The drawing under review shows one solid part. Ordinate dimensions are in mm from its lowest x, y, z. Coordinates: 2 decimals unless noted, no trailing zeros. Order: outer loops, then holes, each group sorted by start corner. A loop starts at its lowest first (then second) coordinate and runs counter-clockwise, first axis right, second up. Notation, with made-up numbers: (-34.5, 77.5) - (-28.5, 77.5) arc R27 ccw to (-28.5, 113.5) - close; hole circle Ø10 at (39.25, 50.5). An arc over 180 degrees is marked (long way). Answer in a Markdown table with one row per item.
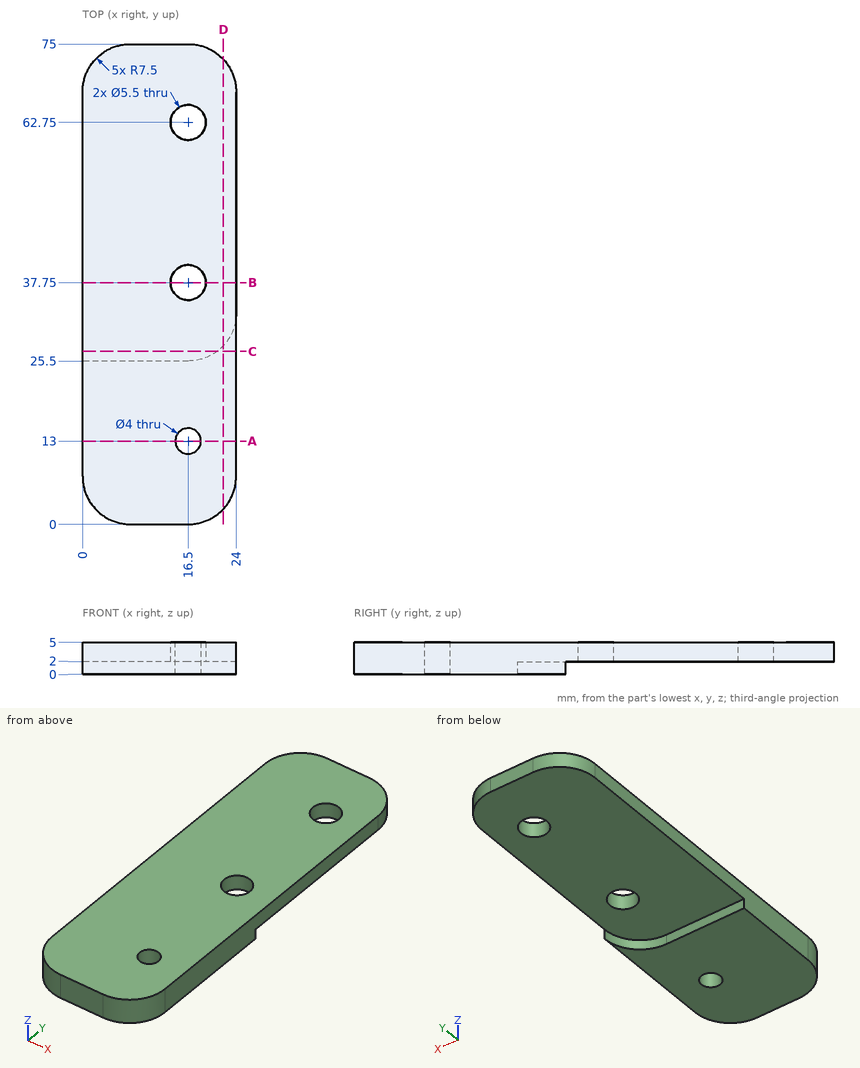
Item 1: Clearance check with flat-ended pins moving along their axes: pin 1 Ø6 at (x, y) = (10.5, 43) entering from -Z; pin 2 Ø0.6 at (x, z) = (6.5, 1.5) entering from +Y; pin 3 Ø3 at (x, z) = (21.5, 1.5) entering from -Y. State where each tip first meets the part, or that it passes through.
Check values:
| item | result |
|---|---|
| pin 1 | z = 2 |
| pin 2 | y = 25.5 |
| pin 3 | y = 0.87 |
Item 2: We need section A-A, the plane y = 13. Write out the cut boundary in (x, z), then the cut area to 3 significant figures.
Check values:
| item | result |
|---|---|
| outline | (0, 0) - (14.5, 0) - (14.5, 5) - (0, 5) - close; (18.5, 0) - (24, 0) - (24, 5) - (18.5, 5) - close |
| area | 100 mm^2 |
Item 3: We need section D-D, the plane x = 22. Write out the cut boundary in (y, z), then the cut area to 3 significant figures.
Check values:
| item | result |
|---|---|
| outline | (2.4, 0) - (27.9, 0) - (27.9, 2) - (72.6, 2) - (72.6, 5) - (2.4, 5) - close |
| area | 262 mm^2 |
Item 4: To check wall thickness, follow line 1 (X direction, y = 62.75, z = 2.75); line 2 (Z direction, x = 3, y = 69.5); line 3 (Y direction, x = 6.75, z = 4.1). State the ranges of each line that lie inside material, in increasing order. Write a range as from..to.
Check values:
| item | result |
|---|---|
| line 1 | 0..13.75, 19.25..24 |
| line 2 | 2..5 |
| line 3 | 0.04..74.96 |
Item 5: We need section C-C, the plane y = 27. Write out the cut boundary in (x, z), then the cut area to 3 significant figures.
Check values:
| item | result |
|---|---|
| outline | (0, 2) - (21, 2) - (21, 0) - (24, 0) - (24, 5) - (0, 5) - close |
| area | 78.0 mm^2 |
Item 6: We need section B-B, the plane y = 37.75. Write out the cut boundary in (x, z), then the cut area to 3 significant figures.
Check values:
| item | result |
|---|---|
| outline | (0, 2) - (13.75, 2) - (13.75, 5) - (0, 5) - close; (19.25, 2) - (24, 2) - (24, 5) - (19.25, 5) - close |
| area | 55.5 mm^2 |
